from build123d import *

# Parameters (mm, degrees)
SKETCH1_W                      = 511.175
SKETCH1_H                      = 127
BASE_FLANGE1_DEPTH             = 1.42875
EDGE_FLANGE1_STRIP_W           = 12.065
EDGE_FLANGE1_STRIP_H           = 1.42875
EDGE_FLANGE1_STRIP_CUT_DEPTH   = 127
EDGE_FLANGE1_STRIP_2_W         = 12.065
EDGE_FLANGE1_STRIP_2_H         = 1.42875
EDGE_FLANGE1_STRIP_CUT_2_DEPTH = 127
EDGE_FLANGE1_DEPTH             = 127
EDGE_FLANGE1_BEND_DEPTH        = 127
CUT_EXTRUDE1_DEPTH             = 534.339544007
FILLET1_R                      = 31.75
SKETCH14_R                     = 14.28115
CUT_EXTRUDE2_DEPTH             = 534.339544007
H_START                        = -255.5875
H_0_266_DIAMETER_SLOT1_DEPTH   = 511.175
F_0_257_DIAMETER_HOLE2_D       = 6.5278
EDGE_FLANGE2_DEPTH             = 501.9675
EDGE_FLANGE2_BEND_DEPTH        = 501.9675


# Read off the part's stored shape, not the designer's step: H (0.266) Diameter Slot1
# Sheet-metal steps are written as plain solids
with BuildPart() as part:
    # Sketch1 → Base-Flange1 (new body)
    with BuildSketch(Plane(origin=(0, 0, 0), x_dir=(1, 0, 0), z_dir=(0, 1, 0))):
        Rectangle(SKETCH1_W, SKETCH1_H)
    extrude(amount=-BASE_FLANGE1_DEPTH)

    # Edge-Flange1 strip (across the edge) → Edge-Flange1 strip cut (cut)
    with BuildSketch(Plane(origin=(255.5875, 0, 63.5), x_dir=(-1, 0, 0), z_dir=(0, 0, -1))):
        with Locations((-1.42875, -0.714375)):
            Rectangle(EDGE_FLANGE1_STRIP_W, EDGE_FLANGE1_STRIP_H)
    extrude(amount=EDGE_FLANGE1_STRIP_CUT_DEPTH, mode=Mode.SUBTRACT)

    # Edge-Flange1 strip 2 (across the edge) → Edge-Flange1 strip cut 2 (cut)
    with BuildSketch(Plane(origin=(-255.5875, 0, -63.5), x_dir=(1, 0, 0), z_dir=(0, 0, 1))):
        with Locations((-1.42875, -0.714375)):
            Rectangle(EDGE_FLANGE1_STRIP_2_W, EDGE_FLANGE1_STRIP_2_H)
    extrude(amount=EDGE_FLANGE1_STRIP_CUT_2_DEPTH, mode=Mode.SUBTRACT)

    # Edge-Flange1 section (across the edge) → Edge-Flange1 (add)
    with BuildSketch(Plane(origin=(255.5875, 0, 63.5), x_dir=(-1, 0, 0), z_dir=(0, 0, -1))):
        with BuildLine():
            Line((0, 3.175), (0, 138.27125))
            Line((0, 138.27125), (1.42875, 138.27125))
            Line((1.42875, 138.27125), (1.42875, 3.175))
            ThreePointArc((1.42875, 3.175), (2.35868597, 0.92993597), (4.60375, 0))
            Line((4.60375, 0), (4.60375, -1.42875))
            ThreePointArc((4.60375, -1.42875), (1.348407156, -0.080342844), (0, 3.175))
        make_face()
    extrude(amount=EDGE_FLANGE1_DEPTH)

    # Edge-Flange1 section 2 (across the edge) → Edge-Flange1 bend (add)
    with BuildSketch(Plane(origin=(-255.5875, 0, -63.5), x_dir=(1, 0, 0), z_dir=(0, 0, 1))):
        with BuildLine():
            Line((0, 3.175), (0, 138.27125))
            Line((0, 138.27125), (1.42875, 138.27125))
            Line((1.42875, 138.27125), (1.42875, 3.175))
            ThreePointArc((1.42875, 3.175), (2.35868597, 0.92993597), (4.60375, 0))
            Line((4.60375, 0), (4.60375, -1.42875))
            ThreePointArc((4.60375, -1.42875), (1.348407156, -0.080342844), (0, 3.175))
        make_face()
    extrude(amount=EDGE_FLANGE1_BEND_DEPTH)

    # Sketch13 → Cut-Extrude1 (cut, through all)
    with BuildSketch(Plane(origin=(255.5875, 0, 0), x_dir=(0, 0, -1), z_dir=(1, 0, 0))):
        Polygon((-63.5, 36.67125), (0, 138.27125), (-63.5, 138.27125), align=None)
    extrude(amount=-CUT_EXTRUDE1_DEPTH, mode=Mode.SUBTRACT)

    # Fillet1
    fillet1_edges = [part.edges().sort_by_distance(p)[0] for p in [
        (254.873125, 138.27125, -63.5),
        (-254.873125, 138.27125, -63.5),
        (254.873125, 138.27125, 0),
        (254.873125, 36.67125, 63.5),
        (-254.873125, 138.27125, 0),
        (-254.873125, 36.67125, 63.5),
    ]]
    fillet(fillet1_edges, radius=FILLET1_R)

    # Sketch14 → Cut-Extrude2 (cut, through all)
    with BuildSketch(Plane(origin=(255.5875, 0, 0), x_dir=(0, 0, -1), z_dir=(1, 0, 0))):
        with Locations(Location((31.75, 106.52125, 0), (0, 0, 90))):
            Circle(SKETCH14_R)
    extrude(amount=-CUT_EXTRUDE2_DEPTH, mode=Mode.SUBTRACT)

    # H (0.266) Diameter Slot1 outline → H (0.266) Diameter Slot1 (cut)
    with BuildSketch(Plane.YZ.offset(H_START)):
        with BuildLine():
            ThreePointArc((20.99945, -43.0657), (17.62125, -39.6875), (14.24305, -43.0657))
            Line((14.24305, -43.0657), (14.24305, -45.8343))
            ThreePointArc((14.24305, -45.8343), (17.62125, -49.2125), (20.99945, -45.8343))
            Line((20.99945, -45.8343), (20.99945, -43.0657))
        make_face()
        with BuildLine():
            ThreePointArc((20.99945, 45.8343), (17.62125, 49.2125), (14.24305, 45.8343))
            Line((14.24305, 45.8343), (14.24305, 43.0657))
            ThreePointArc((14.24305, 43.0657), (17.62125, 39.6875), (20.99945, 43.0657))
            Line((20.99945, 43.0657), (20.99945, 45.8343))
        make_face()
    extrude(amount=H_0_266_DIAMETER_SLOT1_DEPTH, mode=Mode.SUBTRACT)

    # F (0.257) Diameter Hole2 (through all)
    with Locations(Plane(origin=(0, 0, 0), x_dir=(1, 0, 0), z_dir=(0, 1, 0))):
        with Locations((-25.4, -25.4), (25.4, -25.4)):
            Hole(F_0_257_DIAMETER_HOLE2_D / 2)

    # Edge-Flange2 section (across the edge) → Edge-Flange2 (add)
    with BuildSketch(Plane(origin=(-250.98375, 0, 66.675), x_dir=(0, 0, -1), z_dir=(1, 0, 0))):
        with BuildLine():
            Line((-1.42875, 3.175), (-1.42875, 25.4))
            Line((-1.42875, 25.4), (0, 25.4))
            Line((0, 25.4), (0, 3.175))
            ThreePointArc((0, 3.175), (0.92993597, 0.92993597), (3.175, 0))
            Line((3.175, 0), (3.175, -1.42875))
            ThreePointArc((3.175, -1.42875), (-0.080342844, -0.080342844), (-1.42875, 3.175))
        make_face()
    extrude(amount=EDGE_FLANGE2_DEPTH)

    # Edge-Flange2 section 2 (across the edge) → Edge-Flange2 bend (add)
    with BuildSketch(Plane(origin=(250.98375, 0, -66.675), x_dir=(0, 0, 1), z_dir=(-1, 0, 0))):
        with BuildLine():
            Line((-1.42875, 3.175), (-1.42875, 25.4))
            Line((-1.42875, 25.4), (0, 25.4))
            Line((0, 25.4), (0, 3.175))
            ThreePointArc((0, 3.175), (0.92993597, 0.92993597), (3.175, 0))
            Line((3.175, 0), (3.175, -1.42875))
            ThreePointArc((3.175, -1.42875), (-0.080342844, -0.080342844), (-1.42875, 3.175))
        make_face()
    extrude(amount=EDGE_FLANGE2_BEND_DEPTH)


solid = part.part
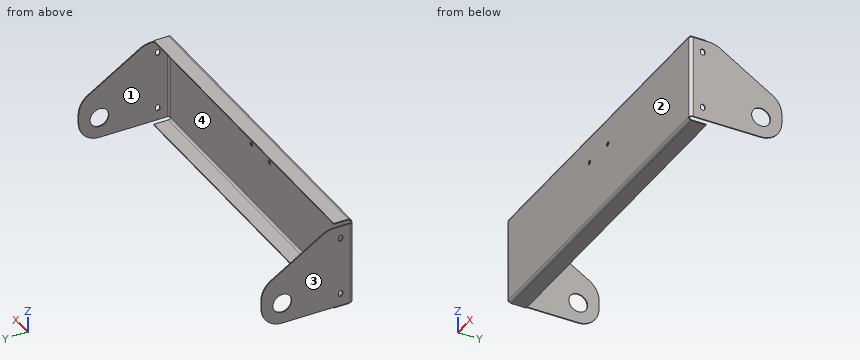
Geometry check sheet. Reference: the model listing, model coordinates, mm. Face numbers are marked on the shaded views. A direction names the side the tool comes from. Give positions to 0.01 mm unless a question says otherwise; leave off trailing zeros. Loops run counter-clockwise (first coordinate to the right, second up) from the corner with the lowest first, then second, coordinate; pieces in that order, holes last. Notation, with made-up numbers: (78, 77) -> (129, 77) arc R13 cw to (129, 94) -> close; hole circle Ø3 at (-31.75, 24.25). An arc over 180 degrees is marked (long way). Answer in a Markdown table with one row per item. Add a question column.
1) Cross-section at A-A on y = 61. Record the boundary of the cut face in (x, z).
2) Gauge pin test, flat ends, axial feed: P1, Ø6, axis at x = -1, z = 52, coming from the +Y side; P2, Ø3.5, axis at x = 254.5, y = 38.5, coming from the -Z side; P3, Ø1.4, axis at x = -253, y = 19, coming from the +Z side; P4, Ø1.1, axis at x = -51, z = 67, coming from the +Y side. Record the tip position at first contact, or that the pin passes through.
3) Set-up check for the marked faces 1 and 2: record each of +Z, -Z, +X, -X, +Y, -Y from which the full face is reachable in a straight line by a thin tool's end or side.
4) Cross-section at D-D on y = 87. Record the boundary of the cut face in (x, z).
5) Material ranges on probe 1 along X at (y, z) = (12, -59); probe 2 along X at (y, z) = (-0.8, 25.4); probe 3 along Z at (x, y) = (171, 24) (3 decimals), recorded low to high. Write a range as from..to.
6) Draft check along Z on the marked faces 3 and 4. Enter one of: pulls with the +Z half, pulls with the -Z half, needs draft (parallel to the pull), parting line crosses it, or undercut.
Outcome:
| question | item | result |
|---|---|---|
| 1 | outline | (-255.59, -63.5) -> (-254.16, -63.5) -> (-254.16, 48.29) -> (-255.59, 48.29) -> close; (254.16, -63.5) -> (255.59, -63.5) -> (255.59, 48.29) -> (254.16, 48.29) -> close |
| 2 | P1 | stops at y = 0 |
| 2 | P2 | stops at z = -63.5 |
| 2 | P3 | passes through |
| 2 | P4 | stops at y = 25.4 |
| 3 | face 1 | +Z, -Z, +Y |
| 3 | face 2 | +Z, -Z, +X, -X, -Y |
| 4 | outline | (-255.59, -63.5) -> (-254.16, -63.5) -> (-254.16, 32.04) -> (-255.59, 32.04) -> close; (254.16, -63.5) -> (255.59, -63.5) -> (255.59, 32.04) -> (254.16, 32.04) -> close |
| 5 | probe 1 | x = -255.59..-254.16, 254.16..255.59 |
| 5 | probe 2 | x = -253.31..-28.66, -22.14..22.14, 28.66..253.31 |
| 5 | probe 3 | z = -68.104..-66.675, 66.675..68.104 |
| 6 | face 3 | needs draft |
| 6 | face 4 | undercut |
